Build history of the part. All positions in model axes, mm. Face numbers are marked on the shaded views. A direction names the side the tool comes from. Round coordinates to 2 decimals unless told otherwise and drop trailing zeros. Order: outer loops, then holes, each group sorted by start corner. A loop starts at its lowest first (then second) coordinate and runs counter-clockwise, first axis right, second up. Notation, with made-up numbers: (-37, 18.25) -> (-15, 18.25) arc R12 cw to (-15, 32.25) -> close; hole circle Ø9 at (-19, 83). An arc over 180 degrees is marked (long way). Answer as CSV lines item,"result". Start each with the question number.
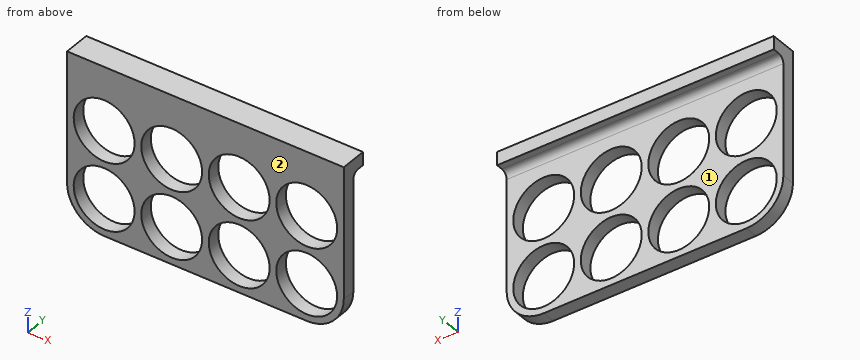
```python
from build123d import *

# Parameters (mm, degrees)
SKETCH1_R           = 9.2
BOSS_EXTRUDE1_DEPTH = 4
SKETCH2_W           = 83.6
SKETCH2_H           = 4
BOSS_EXTRUDE2_DEPTH = 4
FILLET1_R           = 2


with BuildPart() as part:
    # Sketch1 → Boss-Extrude1 (new body)
    with BuildSketch(Plane(origin=(0, 0, 0), x_dir=(1, 0, 0), z_dir=(0, 1, 0))):
        with BuildLine():
            Line((-11.2, 20.4), (-11.2, -19.2))
            Line((-11.2, -19.2), (72.4, -19.2))
            Line((72.4, -19.2), (72.4, 20.4))
            ThreePointArc((72.4, 20.4), (69.119595949, 28.319595949), (61.2, 31.6))
            Line((61.2, 31.6), (0, 31.6))
            ThreePointArc((0, 31.6), (-7.919595949, 28.319595949), (-11.2, 20.4))
        make_face()
        with Locations(Location((0, 0, 0), (0, 0, 270))):
            Circle(SKETCH1_R, mode=Mode.SUBTRACT)
        with Locations(Location((20.4, 0, 0), (0, 0, 270))):
            Circle(SKETCH1_R, mode=Mode.SUBTRACT)
        with Locations(Location((40.8, 0, 0), (0, 0, 270))):
            Circle(SKETCH1_R, mode=Mode.SUBTRACT)
        with Locations(Location((61.2, 0, 0), (0, 0, 270))):
            Circle(SKETCH1_R, mode=Mode.SUBTRACT)
        with Locations(Location((20.4, 20.4, 0), (0, 0, 270))):
            Circle(SKETCH1_R, mode=Mode.SUBTRACT)
        with Locations(Location((40.8, 20.4, 0), (0, 0, 270))):
            Circle(SKETCH1_R, mode=Mode.SUBTRACT)
        with Locations(Location((61.2, 20.4, 0), (0, 0, 270))):
            Circle(SKETCH1_R, mode=Mode.SUBTRACT)
        with Locations(Location((0, 20.4, 0), (0, 0, 270))):
            Circle(SKETCH1_R, mode=Mode.SUBTRACT)
    extrude(amount=BOSS_EXTRUDE1_DEPTH)

    # Sketch2 → Boss-Extrude2 (add)
    with BuildSketch(Plane(origin=(0, 4, 0), x_dir=(1, 0, 0), z_dir=(0, 1, 0))):
        with Locations((30.6, -17.2)):
            Rectangle(SKETCH2_W, SKETCH2_H)
    extrude(amount=BOSS_EXTRUDE2_DEPTH)

    # Fillet1
    fillet1_edges = [part.edges().sort_by_distance(p)[0] for p in [
        (30.6, 4, 15.2),
    ]]
    fillet(fillet1_edges, radius=FILLET1_R)


solid = part.part
```
Q1. Slice it at D-D, the plane z = -12.5. Write the cut outline in (x, y), plus the area to 3 significant figures.
Q2. Slice it at A-A, the plane z = 0. Write the cut outline in (x, y), plus the area to 3 significant figures.
Q3. Slice it at C-C, the plane y = 2.75. Count the separate pieces of the cut face and the enclosed holes in it, plus the area to 3 significant figures.
Q4. Which spindle directions (+Z, -Z, +X, -X, +Y, -Y) get a long thin tool onto all of the face, cutting with end or side? Do the marked faces 1 and 2. Say none if no direction does.
Q5. Probe L1, parallel to X at y = 2.95, z = -20.4; L2, parallel to Z at x = 63, y = 2.25; L3, parallel to Z at x = 21.5, y = 1.25. List the from-to ranges inside material, lowest first.
Q6. Flat gauge pins, fed straight in: pin 1 Ø12 at (x, z) = (7.5, -14) entering from +Y; pin 2 Ø4 at (y, z) = (7, -8) entering from -X; pin 3 Ø2 at (x, y) = (19, 7) entering from -Z; pin 4 Ø10 at (x, z) = (54.5, 9.5) entering from +Y. Where does each tip first touch, or does it go through?
Q7. Slice it at B-B, the plane x = 20.4. Write the cut outline in (y, z).
Solutions:
1,outline,"(-11.2, 0) -> (-4.71, 0) -> (-4.71, 4) -> (-11.2, 4) -> close; (4.71, 0) -> (15.69, 0) -> (15.69, 4) -> (4.71, 4) -> close; (25.11, 0) -> (36.09, 0) -> (36.09, 4) -> (25.11, 4) -> close; (45.51, 0) -> (56.49, 0) -> (56.49, 4) -> (45.51, 4) -> close; (65.91, 0) -> (72.4, 0) -> (72.4, 4) -> (65.91, 4) -> close"
1,area,"184 mm2"
2,outline,"(-11.2, 0) -> (-9.2, 0) -> (-9.2, 4) -> (-11.2, 4) -> close; (9.2, 0) -> (11.2, 0) -> (11.2, 4) -> (9.2, 4) -> close; (29.6, 0) -> (31.6, 0) -> (31.6, 4) -> (29.6, 4) -> close; (50, 0) -> (52, 0) -> (52, 4) -> (50, 4) -> close; (70.4, 0) -> (72.4, 0) -> (72.4, 4) -> (70.4, 4) -> close"
2,area,"40.0 mm2"
3,separate pieces,"1"
3,enclosed holes,"8"
3,area,"2,070 mm2"
4,face 1,"-Z, +X, -X, +Y"
4,face 2,"+Z, -Z, +X, -X, -Y"
5,L1,"x = -11.2 to -9.2, 9.2 to 11.2, 29.6 to 31.6, 50 to 52, 70.4 to 72.4"
5,L2,"z = -31.45 to -29.42, -11.38 to -9.02, 9.02 to 19.2"
5,L3,"z = -31.6 to -29.53, -11.27 to -9.13, 9.13 to 19.2"
6,pin 1,"stops at y = 4"
6,pin 2,"passes through"
6,pin 3,"stops at z = 15.2"
6,pin 4,"stops at y = 4.48"
7,outline,"(0, -31.6) -> (4, -31.6) -> (4, -29.6) -> (0, -29.6) -> close; (0, -11.2) -> (4, -11.2) -> (4, -9.2) -> (0, -9.2) -> close; (0, 9.2) -> (4, 9.2) -> (4, 13.2) arc R2 cw to (6, 15.2) -> (8, 15.2) -> (8, 19.2) -> (0, 19.2) -> close"
